The model under review builds one solid part; all positions refer to its coordinate system, in mm. Face numbers are marked on the shaded views. Coordinates: 2 decimals unless noted, no trailing zeros. Write each loop counter-clockwise with the first axis right and the second up, starting at its lowest first coordinate (ties: lowest second). Pieces come first, ordered by that corner, then holes. Notation, with made-up numbers: (59, -36.5) - (82, -36.5) arc R14 cw to (82, -16.5) - close; hole circle Ø7 at (31, 30.5). An arc over 180 degrees is marked (long way). Return JSON: item names as keys, results as strings. Group by question number.
(1) We need section B-B on x = 0. State the section outline as (y, z) points (3 decimals), then the cut area to 3 significant figures.
(2) We need section A-A on z = 0. State the section outline as (x, y) points (3 decimals).
(3) Draft analysis for pull direction Z (two halves, no side actions). For the marked faces 1 and 2, state which applies: released by +Z, released by -Z, zero draft, split by the parting line, or undercut.
(4) For pin 1 Ø6 at (x, y) = (-47, 10) entering from +Z; pin 2 Ø8 at (x, z) = (89, 47.5) entering from -Y; pin 3 Ø1 at (x, y) = (-21.5, 10.5) entering from +Z, all flat-tipped, find the tip position at first contact; note any pin that passes through.
(5) We need section C-C on y = 10.25. State the section outline as (x, z) points.
(6) To check wall thickness, follow L1, parallel to Y at x = 94.5, z = 23.5; L2, parallel to X at y = 1, z = -74; L3, parallel to X at y = 1.15, z = 0 (3 decimals). State the ranges of each line that lie inside material, in increasing order. Write a range as from..to.
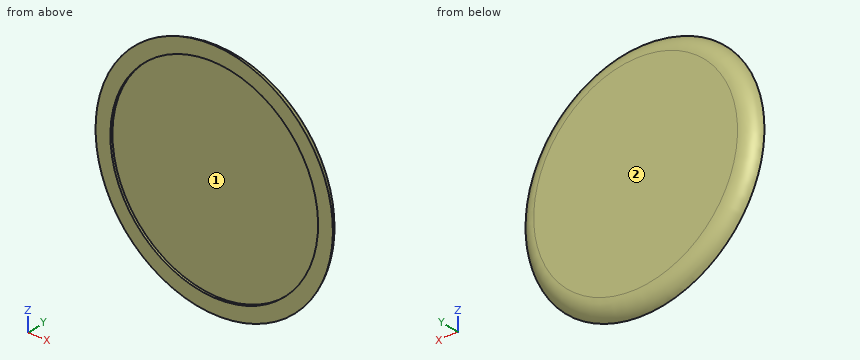
```python
from build123d import *

# Parameters (mm, degrees)
SKETCH2_R           = 127
BOSS_EXTRUDE1_DEPTH = 12.7
FILLET1_R           = 19.05
SKETCH3_R           = 111.125
CUT_EXTRUDE1_DEPTH  = 2.54


with BuildPart() as part:
    # Sketch2 → Boss-Extrude1 (new body)
    with BuildSketch(Plane(origin=(0, 0, 0), x_dir=(1, 0, 0), z_dir=(0, 1, 0))):
        with Locations(Location((0, 0, 0), (0, 0, 270))):
            Circle(SKETCH2_R)
    extrude(amount=BOSS_EXTRUDE1_DEPTH)

    # Fillet1
    # the kernel refuses this fillet: 19.05 mm, written as the material it takes off along each edge
    with BuildSketch(Plane(origin=(0, 12.7, 0), x_dir=(0, 0, 1), z_dir=(-1, 0, 0))) as fillet1_piece_1:
        with BuildLine():
            CenterArc((109.039487758, -19.05), FILLET1_R, 19.471220634, 70.528779366)
            Line((109.039487758, 0), (109.039487758, 0.381))
            Line((109.039487758, 0.381), (127, 0.381))
            Line((127, 0.381), (127.381, 0))
            ThreePointArc((127.381, 0), (127.381, -6.35), (127.359210245, -12.573))
            Line((127.359210245, -12.573), (127, -12.7))
        make_face()
    revolve(axis=Axis((0, 12.7, 0), (0, 1, 0)), mode=Mode.SUBTRACT)

    # Sketch3 → Cut-Extrude1 (cut)
    with BuildSketch(Plane.XZ):
        with Locations(Location((0, 0, 0), (0, 0, 270))):
            Circle(SKETCH3_R)
    extrude(amount=-CUT_EXTRUDE1_DEPTH, mode=Mode.SUBTRACT)


solid = part.part
```
Ans:
{
 "1": {"outline": "(0, -127) arc R19.05 ccw to (12.7, -109.039) - (12.7, 109.039) arc R19.05 ccw to (0, 127) - (0, 111.125) - (2.54, 111.125) - (2.54, -111.125) - (0, -111.125) - close", "area": "2,540 mm²"},
 "2": {"outline": "(-127, 0) - (-111.125, 0) - (-111.125, 2.54) - (111.125, 2.54) - (111.125, 0) - (127, 0) arc R19.05 ccw to (109.039, 12.7) - (-109.039, 12.7) arc R19.05 ccw to start"},
 "3": {"face 1": "undercut", "face 2": "zero draft"},
 "4": {"pin 1": "z = 113.49", "pin 2": "y = 2.54", "pin 3": "z = 116.86"},
 "5": {"outline": "circle Ø236.77 at (0, 0)"},
 "6": {"L1": "2.54..12.7", "L2": "-102.74..-82.9, 82.9..102.74", "L3": "-126.551..-111.125, 111.125..126.551"}
}
